```python
from build123d import *

# Parameters (mm, degrees)
SKETCH_1_R          = 50
EXTRUDE_1_DEPTH     = 20
CUT_EXTRUDE_START   = -18
SKETCH_2_R          = 50
SKETCH_2_R_2        = 47.5
CUT_EXTRUDE_1_DEPTH = 16
SKETCH_3_R          = 6
CUT_EXTRUDE_2_DEPTH = 74.484692283
CHAMFER_1_SIZE      = 0.5
SKETCH_4_W          = 4
SKETCH_4_H          = 8.342964167
CUT_EXTRUDE_3_DEPTH = 74.484692283


with BuildPart() as part:
    # 草图1 → 凸台-拉伸1 (new body)
    with BuildSketch(Plane(origin=(0, 0, 0), x_dir=(1, 0, 0), z_dir=(0, 1, 0))):
        with Locations(Location((0, 0, 0), (0, 0, 270))):
            Circle(SKETCH_1_R)
    extrude(amount=EXTRUDE_1_DEPTH)

    # 草图2 → 切除-拉伸1 (cut)
    with BuildSketch(Plane(origin=(0, 20, 0), x_dir=(1, 0, 0), z_dir=(0, 1, 0)).offset(CUT_EXTRUDE_START)):
        with Locations(Location((0, 0, 0), (0, 0, 270))):
            Circle(SKETCH_2_R)
        with Locations(Location((0, 0, 0), (0, 0, 270))):
            Circle(SKETCH_2_R_2, mode=Mode.SUBTRACT)
    extrude(amount=CUT_EXTRUDE_1_DEPTH, mode=Mode.SUBTRACT)

    # 草图3 → 切除-拉伸2 (cut, through all)
    with BuildSketch(Plane(origin=(0, 20, 0), x_dir=(1, 0, 0), z_dir=(0, 1, 0))):
        with Locations(Location((0, 0, 0), (0, 0, 270))):
            Circle(SKETCH_3_R)
    extrude(amount=-CUT_EXTRUDE_2_DEPTH, mode=Mode.SUBTRACT)

    # 倒角1
    chamfer_1_edges = [part.edges().sort_by_distance(p)[0] for p in [
        (0, 0, -6),
        (0, 20, -6),
    ]]
    chamfer(chamfer_1_edges, length=CHAMFER_1_SIZE)

    # 草图4 → 切除-拉伸3 (cut, through all)
    with BuildSketch(Plane(origin=(0, 20, 0), x_dir=(1, 0, 0), z_dir=(0, 1, 0))):
        with Locations((0, 3.828517917)):
            Rectangle(SKETCH_4_W, SKETCH_4_H)
    extrude(amount=-CUT_EXTRUDE_3_DEPTH, mode=Mode.SUBTRACT)


solid = part.part
```
Could you check a few things on this model? Use its own coordinates, in mm. A direction names the side the tool comes from. Coordinates: 2 decimals unless noted, no trailing zeros. Write each loop counter-clockwise with the first axis right and the second up, starting at its lowest first coordinate (ties: lowest second). Pieces come first, ordered by that corner, then holes. Notation, with made-up numbers: (61, 21.25) -> (97, 21.25) arc R25 cw to (97, 54.25) -> close; hole circle Ø10 at (74.25, -5). An arc over 180 degrees is marked (long way). Write item = value, one per line. Start each with the question number.
(1) I need wall thicknesses on line 1 (X direction, y = 7, z = 0); line 2 (Y direction, x = -23, z = -42); line 3 (Z direction, x = -3, y = 4). Which ranges of each line are inside material? Lowest first, please. Write a range as [from, to].
(2) Will these pins go through, and if not, where does the flat tip stop? pin 1 (3 mm diameter, centred on x = 0.5, y = 6.5, fed in from +Z); pin 2 (1.5 mm diameter, centred on y = 12, z = 17.5, fed in from -X); pin 3 (4 mm diameter, centred on x = -11.5, y = 15, fed in from +Z).
(3) I want a section at A-A (z = 0). Please give me the cut outline in (x, y), plus the area to 3 significant figures.
(4) Which directions (+Z, -Z, +X, -X, +Y, -Y) give clear straight access to the entire face, cutting with the end or side of a thin tool? Please do faces 4 (the face through (-18.3, 18, 44.2)), 5 (the face through (-10, 20, -1)), 6 (the face through (2, 10, -7)).
(5) I want a section at B-B (x = 0). Please give me the cut outline in (y, z), plus the area to 3 significant figures.
(6) I want a section at C-C (y = 5.25). Please give me the cut outline in (x, z), plus the area to 3 significant figures.
(7) We'd pull the mould along Y, two halves only. Please class faces 1 (the face through (-0.243, 19.642, 6.138)), 2 (the face through (-2, 10, -7)), 3 (the face through (-46.37, 9.89, -10.3)): released by +Y, released by -Y, zero draft, split by the parting line, or undercut.
(8) I want a section at D-D (z = -11.5). Please give me the cut outline in (x, y), plus the area to 3 significant figures.
Result set:
q1.line_1 = [-47.5, -6], [6, 47.5]
q1.line_2 = [0, 2], [18, 20]
q1.line_3 = [-47.41, -5.2], [5.2, 47.41]
q2.pin_1 = 47.5
q2.pin_2 = -44.45
q2.pin_3 = 46.54
q3.outline = (-50, 0) -> (-6.5, 0) -> (-6, 0.5) -> (-6, 19.5) -> (-6.5, 20) -> (-50, 20) -> (-50, 18) -> (-47.5, 18) -> (-47.5, 2) -> (-50, 2) -> close; (6, 0.5) -> (6.5, 0) -> (50, 0) -> (50, 2) -> (47.5, 2) -> (47.5, 18) -> (50, 18) -> (50, 20) -> (6.5, 20) -> (6, 19.5) -> close
q3.area = 1,680 mm2
q4.face_4 = none
q4.face_5 = +Z, -Z, +X, -X, +Y
q4.face_6 = +Y, -Y
q5.outline = (0, -50) -> (2, -50) -> (2, -47.5) -> (18, -47.5) -> (18, -50) -> (20, -50) -> (20, -8) -> (0, -8) -> close; (0, 6.5) -> (0.5, 6) -> (19.5, 6) -> (20, 6.5) -> (20, 50) -> (18, 50) -> (18, 47.5) -> (2, 47.5) -> (2, 50) -> (0, 50) -> close
q5.area = 1,640 mm2
q6.outline = circle Ø95 at (0, 0); hole (-2, -8) -> (2, -8) -> (2, -5.66) arc R6 ccw (long way) to (-2, -5.66) -> close
q6.area = 6,970 mm2
q7.face_1 = released by +Y
q7.face_2 = zero draft
q7.face_3 = undercut
q8.outline = (-48.66, 0) -> (48.66, 0) -> (48.66, 2) -> (46.09, 2) -> (46.09, 18) -> (48.66, 18) -> (48.66, 20) -> (-48.66, 20) -> (-48.66, 18) -> (-46.09, 18) -> (-46.09, 2) -> (-48.66, 2) -> close
q8.area = 1,860 mm2
